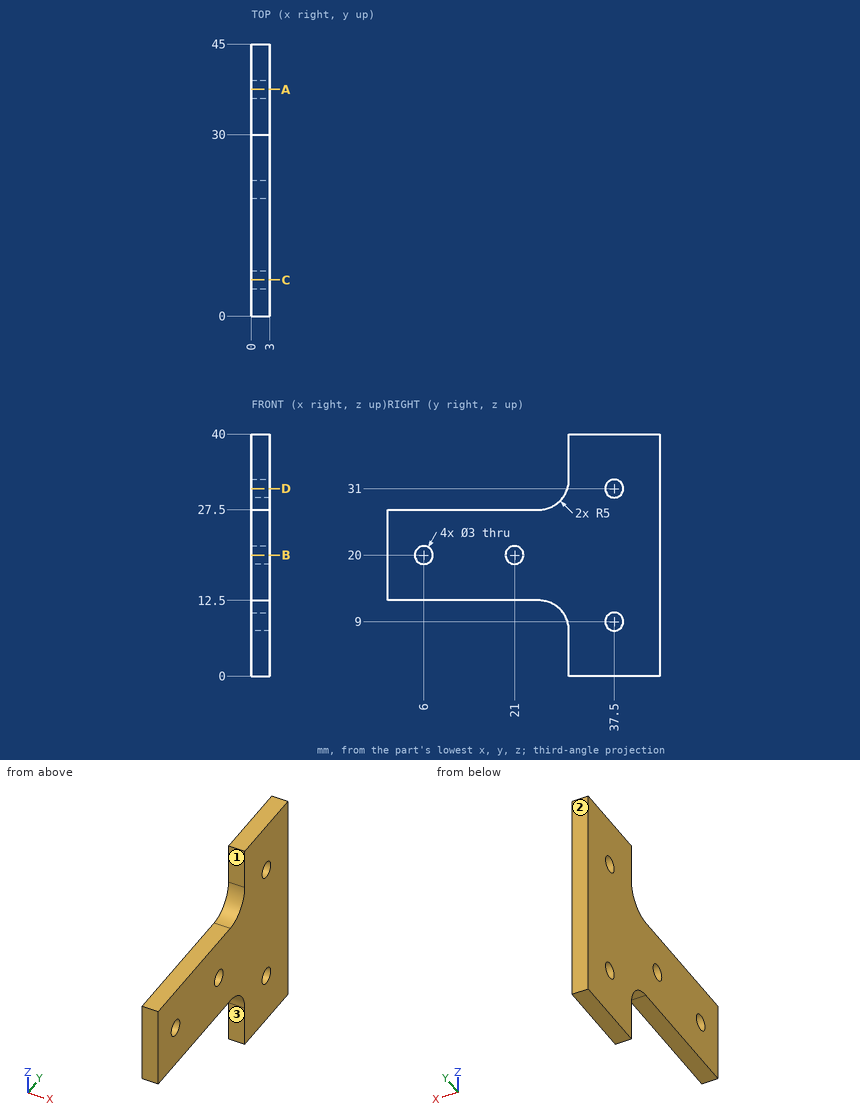
Verification items for this drawing (mm, ordinates from the low corner). A direction names the side the tool comes from. Round coordinates to 2 decimals unless told otherwise and drop trailing zeros. Order: outer loops, then holes, each group sorted by start corner. A loop starts at its lowest first (then second) coordinate and runs counter-clockwise, first axis right, second up. Notation, with made-up numbers: (-19, 66) -> (8, 66) arc R12 cw to (8, 84) -> close; hole circle Ø1 at (44, 44.5). An arc over 180 degrees is marked (long way). Use one line per item in the form item = value.
1. Cross-section at B-B, the plane z = 20. Enter the section's corners in (x, y).
Working result:
outline = (0, 0) -> (3, 0) -> (3, 4.5) -> (0, 4.5) -> close; (0, 7.5) -> (3, 7.5) -> (3, 19.5) -> (0, 19.5) -> close; (0, 22.5) -> (3, 22.5) -> (3, 45) -> (0, 45) -> close
2. Go/stop test with flat-tipped pins: pin 1 (1.5 mm diameter, centred on x = 1.5, y = 18.5, fed in from +Z); pin 2 (1.5 mm diameter, centred on x = 1.5, z = 3, fed in from -Y); pin 3 (2.5 mm diameter, centred on y = 37.5, z = 9, fed in from +X); pin 4 (0.9 mm diameter, centred on x = 1.5, y = 8, fed in from -Z). Record where each tip stops, or that it passes through.
Working result:
pin_1 = 27.5
pin_2 = 30
pin_3 = through
pin_4 = 12.5
3. Cross-section at A-A, the plane y = 37.5. Enter the section's corners in (x, z), plus the area to 3 significant figures.
Working result:
outline = (0, 0) -> (3, 0) -> (3, 7.5) -> (0, 7.5) -> close; (0, 10.5) -> (3, 10.5) -> (3, 29.5) -> (0, 29.5) -> close; (0, 32.5) -> (3, 32.5) -> (3, 40) -> (0, 40) -> close
area = 102 mm^2
4. Set-up check for the marked faces 1, 2 and 3: record each of +Z, -Z, +X, -X, +Y, -Y from which the full face is reachable in a straight line by a thin tool's end or side.
Working result:
face_1 = +Z, +X, -X, -Y
face_2 = +Z, -Z, +X, -X, +Y
face_3 = -Z, +X, -X, -Y
5. Cross-section at D-D, the plane z = 31. Enter the section's corners in (x, y).
Working result:
outline = (0, 29.77) -> (3, 29.77) -> (3, 36) -> (0, 36) -> close; (0, 39) -> (3, 39) -> (3, 45) -> (0, 45) -> close
6. Cross-section at C-C, the plane y = 6. Enter the section's corners in (x, z).
Working result:
outline = (0, 12.5) -> (3, 12.5) -> (3, 18.5) -> (0, 18.5) -> close; (0, 21.5) -> (3, 21.5) -> (3, 27.5) -> (0, 27.5) -> close
7. Scan lines: line 1 along Y through (x, z) = (2.1, 20); line 2 along Y through (x, z) = (2.5, 21); line 3 along Z through (x, y) = (0.65, 15.5). Record each from-to range of solid material in increasing order. Write a range as from..to.
Working result:
line_1 = 0..4.5, 7.5..19.5, 22.5..45
line_2 = 0..4.88, 7.12..19.88, 22.12..45
line_3 = 12.5..27.5
